from build123d import *

# Parameters (mm, degrees)
ESQUISSE1_R             = 17.5
BOSS_EXTRU_1_DEPTH      = 8.8
ESQUISSE4_R             = 6.373182781
ESQUISSE4_R_2           = 2.35
ENL_V_MAT_EXTRU_1_DEPTH = 12.1
ESQUISSE5_R             = 10.689407939
ESQUISSE5_R_2           = 2.35
ENL_V_MAT_EXTRU_2_DEPTH = 12.1
CONG_1_R                = 1


with BuildPart() as part:
    # Esquisse1 → Boss.-Extru.1 (new body)
    with BuildSketch(Plane.XY):
        with BuildLine():
            Line((-33.5, 2.35), (-21.5, 2.35))
            Line((-21.5, 2.35), (-21.37118387, 2.35))
            ThreePointArc((-21.37118387, 2.35), (-20.203391347, 7.353433082), (-17.881827529, 11.936927755))
            Line((-17.881827529, 11.936927755), (-27.173039727, 19.733180483))
            Line((-27.173039727, 19.733180483), (-24.151937962, 23.333589366))
            Line((-24.151937962, 23.333589366), (-14.860725764, 15.537336637))
            ThreePointArc((-14.860725764, 15.537336637), (20.203391347, -7.353433082), (-21.37118387, -2.35))
            Line((-21.37118387, -2.35), (-21.5, -2.35))
            Line((-21.5, -2.35), (-33.5, -2.35))
            Line((-33.5, -2.35), (-33.5, 2.35))
        make_face()
        Circle(ESQUISSE1_R, mode=Mode.SUBTRACT)
    extrude(amount=BOSS_EXTRU_1_DEPTH)

    # Esquisse4 → Enlèv. mat.-Extru.1 (cut)
    with BuildSketch(Plane(origin=(-25.662488844, 21.533384924, 0), x_dir=(0, 0, 1), z_dir=(-0.766044443, 0.64278761, 0))):
        with Locations((4.4, 0)):
            Circle(ESQUISSE4_R)
        with Locations((4.4, 0)):
            Circle(ESQUISSE4_R_2, mode=Mode.SUBTRACT)
    extrude(amount=-ENL_V_MAT_EXTRU_1_DEPTH, mode=Mode.SUBTRACT)

    # Esquisse5 → Enlèv. mat.-Extru.2 (cut)
    with BuildSketch(Plane.ZY.offset(33.5)):
        with Locations((4.4, 0)):
            Circle(ESQUISSE5_R)
        with Locations((4.4, 0)):
            Circle(ESQUISSE5_R_2, mode=Mode.SUBTRACT)
    extrude(amount=-ENL_V_MAT_EXTRU_2_DEPTH, mode=Mode.SUBTRACT)

    # Congé1
    cong_1_edges = [part.edges().sort_by_distance(p)[0] for p in [
        (-25.662488844, 21.533384924, 2.05),
        (-33.5, 0, 2.05),
    ]]
    fillet(cong_1_edges, radius=CONG_1_R)


solid = part.part
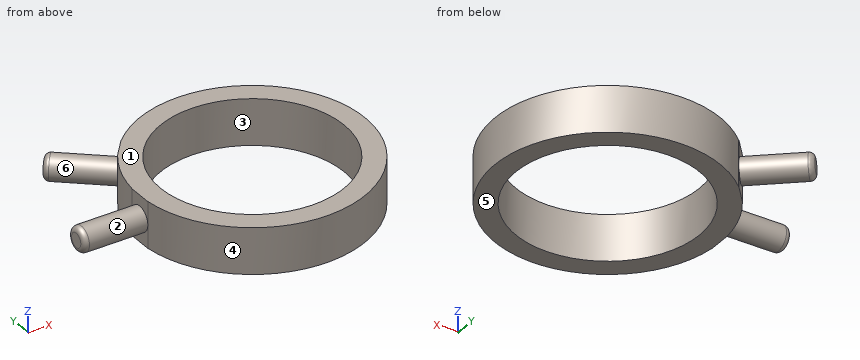
The listing builds one solid part. Answer for the finished solid, in the listing's coordinates (mm). Face numbers are marked on the shaded views. A direction names the side the tool comes from. Coordinates: 2 decimals unless noted, no trailing zeros. Order: outer loops, then holes, each group sorted by start corner. A loop starts at its lowest first (then second) coordinate and runs counter-clockwise, first axis right, second up.
Q1. Given P1, Ø5, axis at x = 5, z = 6.5, coming from the -Y side; P2, Ø8, axis at x = 0.5, y = 11, coming from the -Z side; P3, Ø1.5, axis at y = 16.5, z = 3.5, coming from the +X side, each flat-ended and moving along its own axis, determine where each tip first touches the part or whether it passes through.
Q2. A cutting plane is placed at A-A, the plane y = 0. Write down the section's boundary in (x, z).
Q3. A cutting plane is placed at B-B, the plane x = 0. Write down the section's boundary in (y, z).
Q4. A cutting plane is placed at D-D, the plane x = -28. Write down the section's boundary in (y, z), and give its area (3 significant figures).
Q5. For a pull along Y with two mould halves and no side action, classify the marked faces 3, 4, 5 and 6 as pulls with the +Y half, pulls with the -Y half, needs draft (parallel to the pull), parting line crosses it, or undercut.
Q6. A cutting plane is placed at C-C, the plane x = 7.5. Write down the section's boundary in (y, z), and give its area (3 significant figures).
Q7. Which of the six approach directions +Z, -Z, +X, -X, +Y, -Y give full straight-line access (tool end or side, diameter ignored) to the marked faces 1 and 2?
Q8. Consider line 1 (Y direction, x = 0, z = 2.75); line 2 (Y direction, x = 15, z = 2.5); line 3 (X direction, y = 7, z = 3). Determine where each line is inside the solid, lowest interval first.
Answers follow:
1. P1: stops at y = -21.35
1. P2: passes through
1. P3: stops at x = 14.64
2. outline: (-33.5, 3.05) arc R1 ccw to (-32.5, 2.05) - (-21.4, 2.05) - (-21.4, 0) - (-17.5, 0) - (-17.5, 8.8) - (-21.4, 8.8) - (-21.4, 6.75) - (-32.5, 6.75) arc R1 ccw to (-33.5, 5.75) - close; (17.5, 0) - (21.5, 0) - (21.5, 8.8) - (17.5, 8.8) - close
3. outline: (-21.5, 0) - (-17.5, 0) - (-17.5, 8.8) - (-21.5, 8.8) - close; (17.5, 0) - (21.5, 0) - (21.5, 8.8) - (17.5, 8.8) - close
4. outline: circle Ø4.7 at (0, 4.4)
4. area: 17.3 mm2
5. face 3: undercut
5. face 4: parting line crosses it
5. face 5: needs draft
5. face 6: undercut
6. outline: (-20.15, 0) - (-15.81, 0) - (-15.81, 8.8) - (-20.15, 8.8) - close; (15.81, 0) - (20.15, 0) - (20.15, 8.8) - (15.81, 8.8) - close
6. area: 76.3 mm2
7. face 1: +Z, +X, -X, +Y, -Y
7. face 2: -X
8. line 1: y = -21.5 to -17.5, 17.5 to 21.5
8. line 2: y = -15.4 to -9.01, 9.01 to 15.4
8. line 3: x = -20.33 to -16.04, 16.04 to 20.33
